from build123d import *

# Parameters (mm, degrees)
F0_W     = 290.3982
F0_H     = 228.6
F1_DEPTH = 19.05
F3_DEPTH = 228.601
F4_R     = 85.5
F5_DEPTH = 6.5
F6_R     = 73.5
F7_DEPTH = 12.551
F8_SIZE  = 6.35


with BuildPart() as f1:
    # F0 (on Front) → F1 (new body)
    with BuildSketch(Plane.XZ):
        Rectangle(F0_W, F0_H)
    extrude(amount=F1_DEPTH)

    # F2 (on face) → F3 (cut, through all)
    with BuildSketch(Plane.XY.offset(114.3)):
        Polygon((-134.200577, -19.05), (-145.1991, 0), (-145.1991, -19.05), align=None)
        Polygon((134.200577, 0), (145.1991, -19.05), (145.1991, 0), align=None)
    extrude(amount=-F3_DEPTH, mode=Mode.SUBTRACT)

    # F4 (on face) → F5 (cut)
    with BuildSketch(Plane.XZ.offset(19.05)):
        with Locations((5.499261, 0)):
            Circle(F4_R)
    extrude(amount=-F5_DEPTH, mode=Mode.SUBTRACT)

    # F6 (on face) → F7 (cut, through all)
    with BuildSketch(Plane.XZ.offset(12.55)):
        with Locations((5.499261, 0)):
            Circle(F6_R)
    extrude(amount=-F7_DEPTH, mode=Mode.SUBTRACT)

    # F8
    f8_edges = [f1.edges().sort_by_distance(p)[0] for p in [
        (-68.000739, 0, 0),
    ]]
    chamfer(f8_edges, length=F8_SIZE)


solid = f1.part
Read the model definition and answer for the solid it produces. Units are mm, in the model's axes. A direction names the side the tool comes from. Coordinates: 2 decimals unless noted, no trailing zeros. Loops run counter-clockwise (first coordinate to the right, second up) from the corner with the lowest first, then second, coordinate; pieces in that order, holes last. Notation, with made-up numbers: (66.5, -5) - (74.5, -5) arc R30 ccw to (74.5, 32) - close; hole circle Ø7 at (-14, 31.25). An arc over 180 degrees is marked (long way). Answer in a Markdown table with one row per item.
Q1. Given P1, Ø2, axis at y = -9.5, z = -34.5, coming from the -X side; P2, Ø3, axis at y = -15.5, z = 88.5, coming from the +X side; P3, Ø10, axis at x = -85.5, z = -33, coming from the +Y side; P4, Ø10, axis at y = -15, z = 40, coming from the -X side, each flat-ended and moving along its own axis, determine where each tip first touches the part or whether it passes through.
Here are the results:
| item | result |
|---|---|
| P1 | stops at x = -140.29 |
| P2 | stops at x = 144.02 |
| P3 | stops at y = 0 |
| P4 | stops at x = -139.43 |
Q2. Straight lines are drawn through the part: line 1 along X through (y, z) = (-11.5, -47); line 2 along X through (y, z) = (-12.5, 68); line 3 along Z through (x, y) = (-60.5, -13.5). For each, find the intervals that lie inside material, in ascending order. Write a range as [from, to].
Here are the results:
| item | result |
|---|---|
| line 1 | x = [-138.56, -51.01], [62.01, 140.84] |
| line 2 | x = [-137.98, -22.4], [33.4, 141.42] |
| line 3 | z = [-114.3, -54.35], [54.35, 114.3] |
Q3. The mould has two halves that part along Z. Classify faces 3 (the flat face through (-2, -9, 114.3)), 4 (the flat face through (-139.6, -9.7, 1.6)), 5 (the flat face through (43, -12.55, 64)), 6 (the cylindrical face through (-10.434, -9.493, -71.752)): pulls with the +Z half, pulls with the -Z half, needs draft (parallel to the pull), parting line crosses it, or undercut.
Here are the results:
| item | result |
|---|---|
| face 3 | pulls with the +Z half |
| face 4 | needs draft |
| face 5 | undercut |
| face 6 | undercut |
Q4. Find section A-A on z = 0. Write down the section's boundary in (x, y).
Here are the results:
| item | result |
|---|---|
| outline | (-145.2, 0) - (-134.2, -19.05) - (-80, -19.05) - (-80, -12.55) - (-68, -12.55) - (-68, -6.35) - (-74.35, 0) - close; (79, -12.55) - (91, -12.55) - (91, -19.05) - (145.2, -19.05) - (134.2, 0) - (85.35, 0) - (79, -6.35) - close |
Q5. Find section C-C on z = 93. Write down the section's boundary in (x, y).
Here are the results:
| item | result |
|---|---|
| outline | (-145.2, 0) - (-134.2, -19.05) - (145.2, -19.05) - (134.2, 0) - close |
Q6. For faces 1 (the flat face through (-2, -9, -114.3)), 2 (the cylindrical face through (87.05, -15.85, 25.68)), determine the directions among +Z, -Z, +X, -X, +Y, -Y from which every point of the face is accessible in a straight line to the end or side of a thin tool.
Here are the results:
| item | result |
|---|---|
| face 1 | -Z, +X, -X, +Y, -Y |
| face 2 | -Y |
Q7. Find section B-B on y = -3. Write down the section's boundary in (x, z), plus the area to 3 significant figures.
Here are the results:
| item | result |
|---|---|
| outline | (-143.47, -114.3) - (135.93, -114.3) - (135.93, 114.3) - (-143.47, 114.3) - close; hole circle Ø153.7 at (5.5, 0) |
| area | 45,300 mm^2 |
